```python
from build123d import *

# Parameters (mm, degrees)
FILLET1_R     = 5
FILLET2_R     = 10
CHAMFER1_SIZE = 2


with BuildPart() as part:
    # Sketch1 → Revolve1 (revolve)
    with BuildSketch(Plane.XY, mode=Mode.PRIVATE) as revolve1_sk:
        Polygon((0, 0), (202, 0), (202, 15), (152, 15), (152, 13), (142, 13), (142, 20), (100, 30), (90, 30), (90, 50), (70, 50), (70, 35), (20, 35), (20, 50), (0, 50), align=None)
    revolve(revolve1_sk.sketch.rotate(Axis((0, 0, 0), (1, 0, 0)), 90), axis=Axis((0, 0, 0), (1, 0, 0)))

    # Fillet1
    fillet1_edges = [part.edges().sort_by_distance(p)[0] for p in [
        (90, 0, -30),
    ]]
    fillet(fillet1_edges, radius=FILLET1_R)

    # Fillet2
    fillet2_edges = [part.edges().sort_by_distance(p)[0] for p in [
        (90, 0, -50),
    ]]
    fillet(fillet2_edges, radius=FILLET2_R)

    # Chamfer1
    chamfer1_edges = [part.edges().sort_by_distance(p)[0] for p in [
        (152, 0, -15),
        (202, 0, -15),
    ]]
    chamfer(chamfer1_edges, length=CHAMFER1_SIZE - 0.0001)  # a hair under: the kernel refuses the full size


solid = part.part
```
Here's how the part is built. I have some questions about the finished solid (model axes, mm). A direction names the side the tool comes from. Coordinates: 2 decimals unless noted, no trailing zeros. Loops run counter-clockwise (first coordinate to the right, second up) from the corner with the lowest first, then second, coordinate; pieces in that order, holes last. Notation, with made-up numbers: (66.5, 64.25) - (84.5, 64.25) arc R19 cw to (84.5, 101.25) - close; hole circle Ø6 at (80, -29). An arc over 180 degrees is marked (long way). Return JSON: item names as keys, results as strings. Group by question number.
Item 1: If we section it at D-D on x = 160.5: Write out the boundary of the cut face in (y, z), and give its area (3 significant figures).
Item 2: We'd pull the mould along X, two halves only. Please class faces 4 (the face through (202, 0, 0)), 5 (the face through (74.93, -15.02, 47.69)), 6 (the face through (70, 10, -34)): +X half, -X half, draft (parallel to the pull), parting line (faces both ways), or undercut.
Item 3: On a 3-axis mill with a long thin cutter (end or side, diameter ignored), from which of +Z, -Z, +X, -X, +Y, -Y can I reach the whole of each face in a straight line? I mean faces 1 (the face through (44.65, 34.168, -7.587)), 2 (the face through (9.86, -15.02, 47.69)), 3 (the face through (97.465, -25.296, 16.128)). Say none if no direction works.
Item 4: I need wall thicknesses on line 1 (X direction, y = -36.5, z = -14); line 2 (X direction, y = 17, z = -9); line 3 (X direction, y = 45, z = -4). Which ranges of each line are inside material? Lowest first, please. Write a range as from..to.
Item 5: If we section it at C-C on x = 35: Write out the boundary of the cut face in (y, z), and give its area (3 significant figures).
Item 6: Will these pins go through, and if not, where does the flat tip stop? P1, Ø2, axis at y = -30.5, z = 30.5, coming from the +X side; P2, Ø10, axis at x = 53.5, z = 25, coming from the -Y side; P3, Ø10, axis at y = 17, z = 11.5, coming from the +X side.
Calculated:
{
 "1": {"outline": "circle Ø30 at (0, 0)", "area": "707 mm^2"},
 "2": {"face 4": "+X half", "face 5": "draft", "face 6": "undercut"},
 "3": {"face 1": "none", "face 2": "+X, -X", "face 3": "+X"},
 "4": {"line 1": "x = 0..20, 70..90", "line 2": "x = 0..142", "line 3": "x = 0..20, 70..88.56"},
 "5": {"outline": "circle Ø70 at (0, 0)", "area": "3,850 mm^2"},
 "6": {"P1": "stops at x = 89.77", "P2": "stops at y = -28.72", "P3": "stops at x = 142"}
}
